Verification items for this drawing (mm, ordinates from the low corner). Give positions to 0.01 mm unless a question says otherwise; leave off trailing zeros. Loops run counter-clockwise (first coordinate to the right, second up) from the corner with the lowest first, then second, coordinate; pieces in that order, holes last. Notation, with made-up numbers: M -32.5,33.25 L -6.5,33.25 A23 cw -6.5,50.25 Z; hole C 14.25,-9.75 d6. An arc over 180 degrees is marked long. Put each result on its own line as item: value. Start each with the question number.
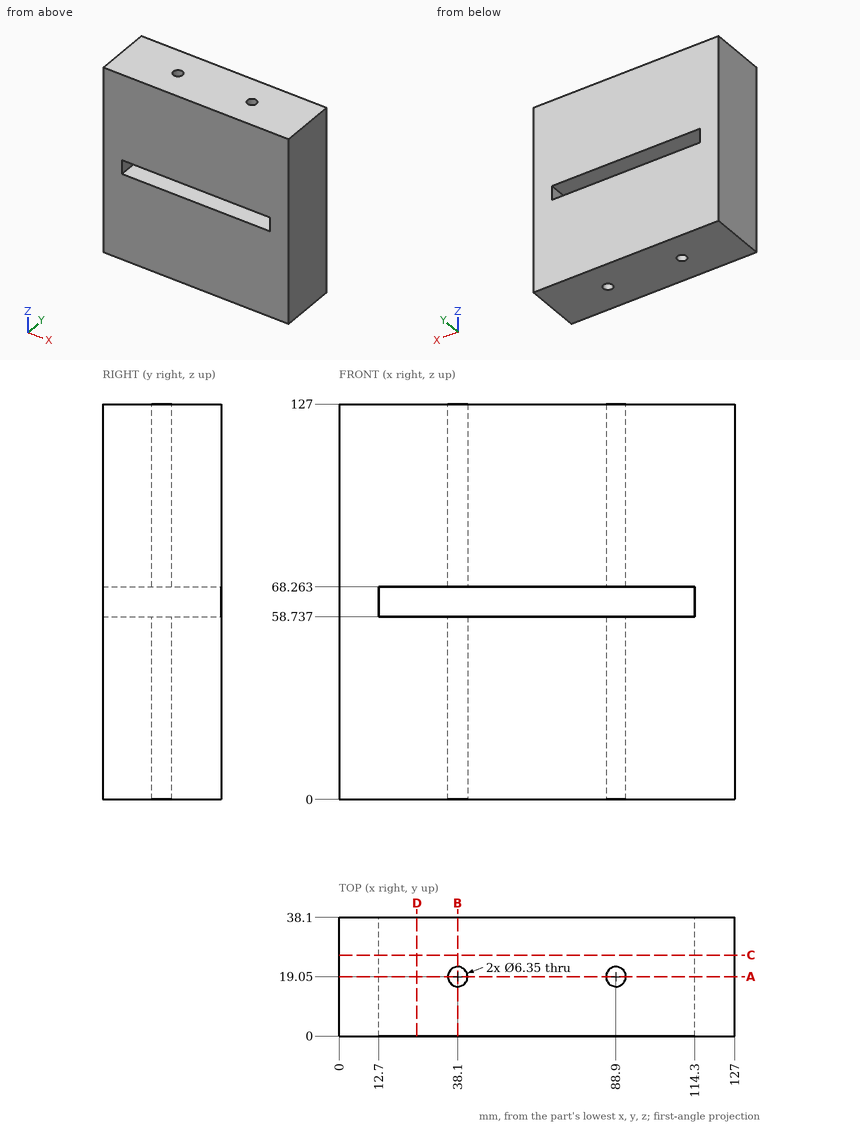
Q1. Cross-section at A-A, the plane y = 19.05. Record the boundary of the cut face in (x, z) (1 decimal).
Q2. Cross-section at D-D, the plane x = 25. Record the boundary of the cut face in (y, z).
Q3. Cross-section at C-C, the plane y = 26. Record the boundary of the cut face in (x, z), then the cut area to 3 significant figures.
Q4. Scan lines: L1, parallel to X at y = 19, z = 102 (1 decimal); L2, parallel to Z at x = 92.5, y = 32.5; L3, parallel to X at y = 18.5, z = 86. Record each from-to range of solid material in increasing order.
Q5. Cross-section at B-B, the plane x = 38.1. Record the boundary of the cut face in (y, z) (1 decimal).
Ans:
1. outline: M 0,0 L 34.9,0 L 34.9,58.7 L 12.7,58.7 L 12.7,68.3 L 34.9,68.3 L 34.9,127 L 0,127 Z; M 41.3,0 L 85.7,0 L 85.7,58.7 L 41.3,58.7 Z; M 41.3,68.3 L 85.7,68.3 L 85.7,127 L 41.3,127 Z; M 92.1,0 L 127,0 L 127,127 L 92.1,127 L 92.1,68.3 L 114.3,68.3 L 114.3,58.7 L 92.1,58.7 Z
2. outline: M 0,0 L 38.1,0 L 38.1,58.74 L 0,58.74 Z; M 0,68.26 L 38.1,68.26 L 38.1,127 L 0,127 Z
3. outline: M 0,0 L 127,0 L 127,127 L 0,127 Z; hole M 12.7,58.74 L 114.3,58.74 L 114.3,68.26 L 12.7,68.26 Z
3. area: 15,200 mm^2
4. L1: x = 0 to 34.9, 41.3 to 85.7, 92.1 to 127
4. L2: z = 0 to 58.74, 68.26 to 127
4. L3: x = 0 to 34.97, 41.23 to 85.77, 92.03 to 127
5. outline: M 0,0 L 15.9,0 L 15.9,58.7 L 0,58.7 Z; M 0,68.3 L 15.9,68.3 L 15.9,127 L 0,127 Z; M 22.2,0 L 38.1,0 L 38.1,58.7 L 22.2,58.7 Z; M 22.2,68.3 L 38.1,68.3 L 38.1,127 L 22.2,127 Z
